```python
from build123d import *

# Parameters (mm, degrees)
BOSS_EXTRUDE1_DEPTH = 2
SKETCH1_5_W         = 22
SKETCH1_5_H         = 91
CUT_EXTRUDE1_DEPTH  = 3


with BuildPart() as part:
    # Sketch1 → Boss-Extrude1 (new body)
    with BuildSketch(Plane.XY):
        Polygon((-99, 90.5), (-99, 7.5), (-90.5, 7.5), (-90.5, -1), (-7.5, -1), (-7.5, 7.5), (1, 7.5), (1, 90.5), (-7.5, 90.5), (-7.5, 99), (-90.5, 99), (-90.5, 90.5), align=None)
    extrude(amount=BOSS_EXTRUDE1_DEPTH)

    # Sketch1<5> → Cut-Extrude1 (cut, through all)
    with BuildSketch(Plane.XY):
        with Locations((-66, 49.5)):
            Rectangle(SKETCH1_5_W, SKETCH1_5_H)
    extrude(amount=CUT_EXTRUDE1_DEPTH, mode=Mode.SUBTRACT)


solid = part.part
```
The listing builds one solid part. Answer for the finished solid, in the listing's coordinates (mm). Round coordinates to 2 decimals unless told otherwise and drop trailing zeros. Write each loop counter-clockwise with the first axis right and the second up, starting at its lowest first coordinate (ties: lowest second). Pieces come first, ordered by that corner, then holes. Notation, with made-up numbers: (27, 35) -> (67, 35) arc R25 ccw to (67, 69) -> close; hole circle Ø11 at (-39.75, 32). An arc over 180 degrees is marked (long way). Answer as a JSON object with one key per item and string values. Group by question number.
Q1. Straight lines are drawn through the part: line 1 along X through (y, z) = (90, 0.3); line 2 along X through (y, z) = (5.5, 1.8); line 3 along Y through (x, z) = (-72, 0.3). For each, find the intervals that lie inside material, in ascending order.
Q2. Section A-A (y = 93) is taken. Write down the section's boundary in (x, z), plus the area to 3 significant figures.
Q3. Section D-D (x = -6) is taken. Write down the section's boundary in (y, z).
Q4. Section C-C (z = 1.65) is taken. Write down the section's boundary in (x, y), plus the area to 3 significant figures.
Q5. Section B-B (x = -61) is taken. Write down the section's boundary in (y, z).
Q6. Each of these flat-tipped pins is pushed along its axis until it touches: pin 1 Ø0.6 at (x, z) = (-2.5, 1) entering from +Y; pin 2 Ø0.6 at (y, z) = (2, 1) entering from -X. Where does it stop, or does it pass through?
Check values:
{
 "1": {"line 1": "-99 to -77, -55 to 1", "line 2": "-90.5 to -77, -55 to -7.5", "line 3": "-1 to 4, 95 to 99"},
 "2": {"outline": "(-90.5, 0) -> (-77, 0) -> (-77, 2) -> (-90.5, 2) -> close; (-55, 0) -> (-7.5, 0) -> (-7.5, 2) -> (-55, 2) -> close", "area": "122 mm^2"},
 "3": {"outline": "(7.5, 0) -> (90.5, 0) -> (90.5, 2) -> (7.5, 2) -> close"},
 "4": {"outline": "(-99, 7.5) -> (-90.5, 7.5) -> (-90.5, -1) -> (-7.5, -1) -> (-7.5, 7.5) -> (1, 7.5) -> (1, 90.5) -> (-7.5, 90.5) -> (-7.5, 99) -> (-90.5, 99) -> (-90.5, 90.5) -> (-99, 90.5) -> close; hole (-77, 4) -> (-55, 4) -> (-55, 95) -> (-77, 95) -> close", "area": "7,710 mm^2"},
 "5": {"outline": "(-1, 0) -> (4, 0) -> (4, 2) -> (-1, 2) -> close; (95, 0) -> (99, 0) -> (99, 2) -> (95, 2) -> close"},
 "6": {"pin 1": "y = 90.5", "pin 2": "x = -90.5"}
}
